Check sheet for the drawn part. Datum: minimum x, y, z corner. Units: mm. Round coordinates to 2 decimals unless told otherwise and drop trailing zeros. Write each loop counter-clockwise with the first axis right and the second up, starting at its lowest first coordinate (ties: lowest second). Pieces come first, ordered by that corner, then holes. Notation, with made-up numbers: (14, -32.75) -> (29, -32.75) arc R15 cw to (29, -4.75) -> close; hole circle Ø4 at (89.25, -14). An arc over 180 degrees is marked (long way). Use a Markdown table: item, result.
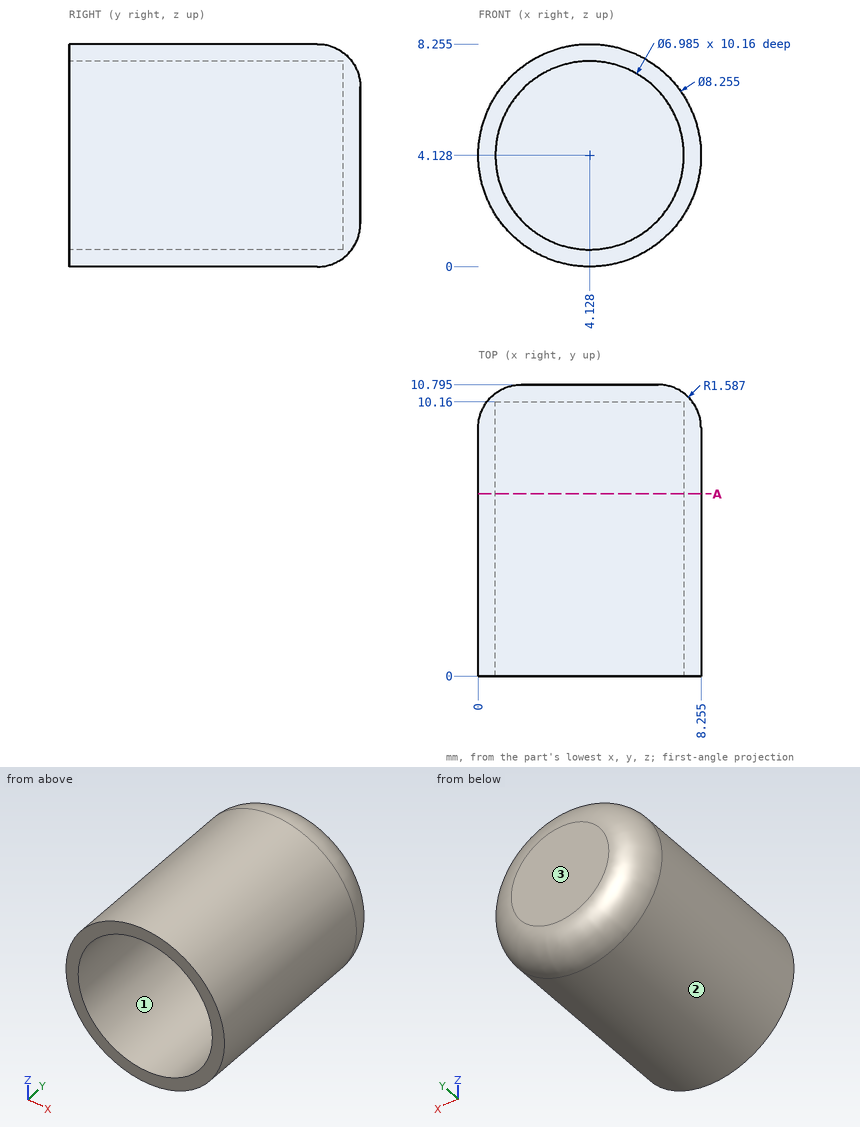
(1) Release check for a two-part mould opening along X. For the marked faces 1, 2 and 3 record: +X half, -X half, draft (parallel to the pull), parting line (faces both ways), or undercut.
A:
| item | result |
|---|---|
| face 1 | undercut |
| face 2 | parting line |
| face 3 | draft |
(2) Section check A-A on y = 6.75. Record the cut outline in (x, z) (1 decimal).
A:
| item | result |
|---|---|
| outline | circle Ø8.3 at (4.1, 4.1); hole circle Ø7 at (4.1, 4.1) |
(3) Thickness scan on line 1 (X direction, y = 1, z = 4.25); line 2 (X direction, y = 6.5, z = 3.5). Record the ranges inside material, lowest first.
A:
| item | result |
|---|---|
| line 1 | x = 0 to 0.64, 7.62 to 8.25 |
| line 2 | x = 0.05 to 0.69, 7.56 to 8.21 |
(4) Gauge pin test, flat ends, axial feed: pin 1 Ø2 at (y, z) = (2.5, 6) entering from +X; pin 2 Ø1 at (x, z) = (2.5, 1) entering from +Y; pin 3 Ø1.5 at (x, y) = (6, 7) entering from +Z. Record the tip position at first contact, or that the pin passes through.
A:
| item | result |
|---|---|
| pin 1 | stops at x = 8.16 |
| pin 2 | stops at y = 10.72 |
| pin 3 | stops at z = 8.1 |
